Could you check a few things on this model? Use its own coordinates, in mm. A direction names the side the tool comes from. Coordinates: 2 decimals unless noted, no trailing zeros. Write each loop counter-clockwise with the first axis right and the second up, starting at its lowest first coordinate (ties: lowest second). Pieces come first, ordered by that corner, then holes.
```python
from build123d import *

# Parameters (mm, degrees)
F0_W      = 45
F0_H      = 45
F1_DEPTH  = 950
F2_R      = 5
F3_W      = 45
F3_H      = 20
F4_DEPTH  = 45.001
F5_W      = 40
F5_H      = 20
F6_DEPTH  = 25
F7_W      = 40
F7_H      = 20
F8_DEPTH  = 25
F9_W      = 575
F9_H      = 20
F10_DEPTH = 230
F11_W     = 575
F11_H     = 30
F12_DEPTH = 10


# Not quite as in the source:
# - a pattern or mirror of a feature is missing from the dataset's text; its kind, count and spacing are read off the source's solid


with BuildPart() as f1:
    # F0 (on Right) → F1 (new body, symmetric)
    with BuildSketch(Plane.YZ):
        with Locations((22.5, 22.5)):
            Rectangle(F0_W, F0_H)
    extrude(amount=F1_DEPTH, both=True)

    # F2
    f2_edges = [f1.edges().sort_by_distance(p)[0] for p in [
        (0, 0, 45),
        (0, 45, 45),
        (0, 0, 0),
        (0, 45, 0),
    ]]
    fillet(f2_edges, radius=F2_R)

    # F3 (on face) → F4 (cut, through all)
    with BuildSketch(Plane.XZ):
        with Locations((-927.5, 22.5)):
            Rectangle(F3_W, F3_H)
    f4 = extrude(amount=-F4_DEPTH, mode=Mode.SUBTRACT)

    # F4_copies: F4 across plane
    add(f4.mirror(Plane(origin=(0, 0, 0), x_dir=(0, 0, 1), z_dir=(1, 0, 0))), mode=Mode.SUBTRACT)

    # F5 (on face) → F6 (cut)
    with BuildSketch(Plane(origin=(0, 0, 0), x_dir=(1, 0, 0), z_dir=(0, 0, -1))):
        with Locations((-780, -22.5)):
            Rectangle(F5_W, F5_H)
    f6 = extrude(amount=-F6_DEPTH, mode=Mode.SUBTRACT)

    # F6_copies: F6 across plane
    add(f6.mirror(Plane(origin=(0, 0, 0), x_dir=(0, 0, 1), z_dir=(1, 0, 0))), mode=Mode.SUBTRACT)

    # F7 (on face) → F8 (cut)
    with BuildSketch(Plane(origin=(0, 0, 0), x_dir=(1, 0, 0), z_dir=(0, 0, -1))):
        with Locations((0, -22.5)):
            Rectangle(F7_W, F7_H)
    extrude(amount=-F8_DEPTH, mode=Mode.SUBTRACT)

    # F9 (on face) → F10 (join)
    with BuildSketch(Plane(origin=(0, 45, 0), x_dir=(-1, 0, 0), z_dir=(0, 1, 0))):
        with Locations((-617.5, 22.5)):
            Rectangle(F9_W, F9_H)
        with Locations((617.5, 22.5)):
            Rectangle(F9_W, F9_H)
    extrude(amount=F10_DEPTH)

    # F11 (on face) → F12 (join)
    with BuildSketch(Plane.XY.offset(32.5)):
        with Locations((-617.5, 260)):
            Rectangle(F11_W, F11_H)
        with Locations((617.5, 260)):
            Rectangle(F11_W, F11_H)
    extrude(amount=F12_DEPTH)


solid = f1.part
```
1. I want a section at A-A on y = 175. Please give me the cut outline in (x, z), plus the area to 3 significant figures.
Verdict:
outline: (-905, 12.5) - (-330, 12.5) - (-330, 32.5) - (-905, 32.5) - close; (330, 12.5) - (905, 12.5) - (905, 32.5) - (330, 32.5) - close
area: 23,000 mm2
2. If we mould it in two halves opening along Z, with no side actions, what happens to faces 6 (the face through (330, 158, 24)), 7 (the face through (13, 11, 0)), 8 (the face through (928, 22, 12.5)), 9 (the face through (-613, 144, 32.5))? For each: pulls with the +Z half, pulls with the -Z half, needs draft (parallel to the pull), parting line crosses it, or undercut.
Verdict:
face 6: needs draft
face 7: pulls with the -Z half
face 8: undercut
face 9: pulls with the +Z half
3. I want a section at B-B on x = -167. Please give me the cut outline in (y, z).
Verdict:
outline: (0, 5) arc R5 ccw to (5, 0) - (40, 0) arc R5 ccw to (45, 5) - (45, 40) arc R5 ccw to (40, 45) - (5, 45) arc R5 ccw to (0, 40) - close
4. For pin 1 (8 mm diameter, centred on x = 575.5, y = 187.5, fed in from +Z); pin 2 (12.5 mm diameter, centred on x = 776.5, z = 10, fed in from +Y); pin 3 (1.5 mm diameter, centred on y = 143, z = 27, fed in from -X); pin 4 (10 mm diameter, centred on y = 206.5, z = 17.5, fed in from +X), each with a flat end and sliding along its axis, tell me the tip position at first contact or that it passes through.
Verdict:
pin 1: stops at z = 32.5
pin 2: stops at y = 275
pin 3: stops at x = -905
pin 4: stops at x = 905
5. On a 3-axis mill with a long thin cutter (end or side, diameter ignored), from which of +Z, -Z, +X, -X, +Y, -Y can I reach the whole of each face in a straight line? I mean faces 1 (the face through (622, 144, 32.5)), 2 (the face through (928, 22, 32.5)), 3 (the face through (613, 260, 42.5)), 4 (the face through (-928, 22, 32.5)), 5 (the face through (-330, 158, 24)). Say none if no direction works.
Verdict:
face 1: +Z, +X, -X
face 2: +X, +Y, -Y
face 3: +Z, +X, -X, +Y
face 4: -X, +Y, -Y
face 5: +Z, -Z, +Y
6. Please list where these lines run through material, in increasing order: line 1 along X through (y, z) = (81, 30); line 2 along X through (y, z) = (23, 11); line 3 along Z through (x, y) = (-826, 114.5).
Verdict:
line 1: x = -905 to -330, 330 to 905
line 2: x = -950 to -800, -760 to -20, 20 to 760, 800 to 950
line 3: z = 12.5 to 32.5
7. I want a section at C-C on x = -400.5. Please give me the cut outline in (y, z).
Verdict:
outline: (0, 5) arc R5 ccw to (5, 0) - (40, 0) arc R5 ccw to (45, 5) - (45, 12.5) - (275, 12.5) - (275, 42.5) - (245, 42.5) - (245, 32.5) - (45, 32.5) - (45, 40) arc R5 ccw to (40, 45) - (5, 45) arc R5 ccw to (0, 40) - close
